Design review of the part built by this model. Coordinates are the model's own, in mm. A direction names the side the tool comes from. Give positions to 0.01 mm unless a question says otherwise; leave off trailing zeros. Order: outer loops, then holes, each group sorted by start corner. A loop starts at its lowest first (then second) coordinate and runs counter-clockwise, first axis right, second up. Notation, with made-up numbers: (38, -33) -> (60, -33) arc R20 ccw to (60, -3) -> close; hole circle Ø4 at (22, 18.25). An arc over 180 degrees is marked (long way). One line per item, written item: value.
from build123d import *

# Parameters (mm, degrees)
SKETCH1_W           = 118
SKETCH1_H           = 50
BOSS_EXTRUDE1_DEPTH = 2
SKETCH2_W           = 5
SKETCH2_H           = 50
BOSS_EXTRUDE2_DEPTH = 6.5
SKETCH3_R           = 1.5
CUT_EXTRUDE1_DEPTH  = 7


with BuildPart() as part:
    # Sketch1 → Boss-Extrude1 (new body)
    with BuildSketch(Plane(origin=(0, 0, 0), x_dir=(1, 0, 0), z_dir=(0, 1, 0))):
        Rectangle(SKETCH1_W, SKETCH1_H)
    extrude(amount=BOSS_EXTRUDE1_DEPTH)

    # Sketch2 → Boss-Extrude2 (add)
    with BuildSketch(Plane(origin=(0, 2, 0), x_dir=(1, 0, 0), z_dir=(0, 1, 0))):
        with Locations((-38.6, 0)):
            Rectangle(SKETCH2_W, SKETCH2_H)
        with Locations((38.6, 0)):
            Rectangle(SKETCH2_W, SKETCH2_H)
    extrude(amount=BOSS_EXTRUDE2_DEPTH)

    # Sketch3 → Cut-Extrude1 (cut)
    with BuildSketch(Plane(origin=(-36.1, 0, 0), x_dir=(0, 0, -1), z_dir=(1, 0, 0))):
        with Locations((-20.34, 5.589776131)):
            Circle(SKETCH3_R)
        with Locations((19.66, 5.6)):
            Circle(SKETCH3_R)
    cut_extrude1 = extrude(amount=-CUT_EXTRUDE1_DEPTH, mode=Mode.SUBTRACT)

    # Mirror1: Cut-Extrude1 across plane
    add(cut_extrude1.mirror(Plane(origin=(0, 0, 0), x_dir=(0, 0, 1), z_dir=(1, 0, 0))), mode=Mode.SUBTRACT)


solid = part.part
Item 1: Machinability: for faces 5 (the flat face through (50, 2, 0)), 6 (the flat face through (-36.1, 5, 0)), 7 (the flat face through (-50, 2, 0)), which of the approach directions +Z, -Z, +X, -X, +Y, -Y give a long, thin tool a straight path to every point of the face, cutting with its end or side? Answer none if there is none.
Returned:
face 5: +Z, -Z, +X, +Y
face 6: +Z, -Z, +Y
face 7: +Z, -Z, -X, +Y
Item 2: Add section C-C on x = 12. Give the boundary of the cut face in (y, z), plus the area to 3 significant figures.
Returned:
outline: (0, -25) -> (2, -25) -> (2, 25) -> (0, 25) -> close
area: 100 mm²
Item 3: Add section B-B on z = -12. Give the boundary of the cut face in (x, y), plus the area to 3 significant figures.
Returned:
outline: (-59, 0) -> (59, 0) -> (59, 2) -> (41.1, 2) -> (41.1, 8.5) -> (36.1, 8.5) -> (36.1, 2) -> (-36.1, 2) -> (-36.1, 8.5) -> (-41.1, 8.5) -> (-41.1, 2) -> (-59, 2) -> close
area: 301 mm²
Item 4: Clearance check with flat-ended pins moving along their axes: P1, Ø5.5, axis at x = -51.5, z = -4, coming from the +Y side; P2, Ø2, axis at y = 6.5, z = 20, coming from the -X side; P3, Ø5, axis at y = 6, z = 11, coming from the +X side. State where each tip first meets the part, or that it passes through.
Returned:
P1: y = 2
P2: x = -41.1
P3: x = 41.1
Item 5: Draft analysis for pull direction X (two halves, no side actions). For faces 1 (the flat face through (36.1, 5, 0)), 2 (the cylindrical face through (38.56, 6.04, 18.91)), 3 (the flat face through (-41.1, 5, 0)), 4 (the flat face through (-1, 2, 0)), state which applies: pulls with the +X half, pulls with the -X half, needs draft (parallel to the pull), parting line crosses it, or undercut.
Returned:
face 1: undercut
face 2: needs draft
face 3: pulls with the -X half
face 4: undercut
Item 6: To check wall thickness, follow line 1 along Z through (x, y) = (37.95, 5.6); line 2 along X through (y, z) = (5.5, -6); line 3 along Y through (x, z) = (-39.5, -19.66). State the ranges of each line that lie inside material, in increasing order. Write a range as from..to.
Returned:
line 1: -25..-21.16, -18.16..18.84, 21.84..25
line 2: -41.1..-36.1, 36.1..41.1
line 3: 0..4.1, 7.1..8.5
Item 7: Add section A-A on z = 20.34. Give the boundary of the cut face in (x, y), plus the area to 3 significant figures.
Returned:
outline: (-59, 0) -> (59, 0) -> (59, 2) -> (41.1, 2) -> (41.1, 4.09) -> (36.1, 4.09) -> (36.1, 2) -> (-36.1, 2) -> (-36.1, 4.09) -> (-41.1, 4.09) -> (-41.1, 2) -> (-59, 2) -> close; (-41.1, 7.09) -> (-36.1, 7.09) -> (-36.1, 8.5) -> (-41.1, 8.5) -> close; (36.1, 7.09) -> (41.1, 7.09) -> (41.1, 8.5) -> (36.1, 8.5) -> close
area: 271 mm²
